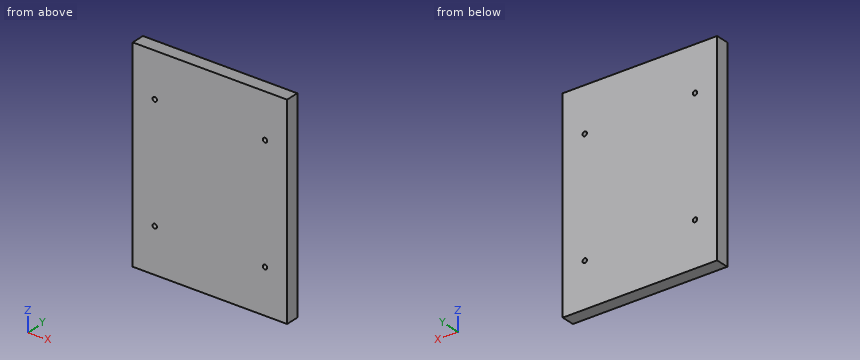
Autodesk Fusion 360 part; units mm, degrees
sketch "Sketch1" plane through (0, 0, 0) normal (0, 1, 0) x (1, 0, 0)
  line L0 (17.5, 23) -> (-17.5, 23)
  line L1 (-17.5, 23) -> (-17.5, -23)
  line L2 (-17.5, -23) -> (17.5, -23)
  line L3 (17.5, -23) -> (17.5, 23)
  line L4 (17.5, 23) -> (-17.5, -23) construction
  line L5 (-17.5, 23) -> (17.5, -23) construction
  circle A0 centre (-12.5, -13) radius 0.5
  circle A1 centre (12.5, -13) radius 0.5
  circle A2 centre (12.5, 13) radius 0.5
  circle A3 centre (-12.5, 13) radius 0.5
  dimension "d1" = 46
  dimension "d2" = 35
  dimension "d3" = 1
  dimension "d4" = 1
  dimension "d5" = 1
  dimension "d6" = 1
  dimension "d7" = 10
  dimension "d8" = 5
  dimension "d9" = 5
  dimension "d10" = 10
  dimension "d11" = 10
  dimension "d12" = 5
  dimension "d13" = 10
  dimension "d14" = 5
  dimension "d15" = 15
  dimension "d16" = 15
extrude "Extrude1" add sketch "Sketch1" along normal blind 3
Geometry check sheet. Reference: the model listing, model coordinates, mm. Coordinates: 2 decimals unless noted, no trailing zeros. Loops run counter-clockwise (first coordinate to the right, second up) from the corner with the lowest first, then second, coordinate; pieces in that order, holes last.
Item 1: Sectioned sample at B-B, the plane z = 13. Record the boundary of the cut face in (x, y).
Item 2: Sectioned sample at A-A, the plane x = -12.5. Record the boundary of the cut face in (y, z), then the cut area to 3 significant figures.
Item 3: Thickness scan on line 1 (Z direction, x = 12.5, y = 2.35); line 2 (X direction, y = 0.85, z = 13). Record the ranges inside material, lowest first.
Check result:
1. outline: (-17.5, 0) - (-13, 0) - (-13, 3) - (-17.5, 3) - close; (-12, 0) - (12, 0) - (12, 3) - (-12, 3) - close; (13, 0) - (17.5, 0) - (17.5, 3) - (13, 3) - close
2. outline: (0, -23) - (3, -23) - (3, -13.5) - (0, -13.5) - close; (0, -12.5) - (3, -12.5) - (3, 12.5) - (0, 12.5) - close; (0, 13.5) - (3, 13.5) - (3, 23) - (0, 23) - close
2. area: 132 mm2
3. line 1: z = -23 to -13.5, -12.5 to 12.5, 13.5 to 23
3. line 2: x = -17.5 to -13, -12 to 12, 13 to 17.5
